Geometry check sheet. Reference: the model listing, model coordinates, mm. A direction names the side the tool comes from. Coordinates: 2 decimals unless noted, no trailing zeros. Loops run counter-clockwise (first coordinate to the right, second up) from the corner with the lowest first, then second, coordinate; pieces in that order, holes last. Notation, with made-up numbers: (-24.5, 49.5) - (22.5, 49.5) arc R30 cw to (22.5, 86.5) - close; hole circle Ø1 at (73, -34). An arc over 180 degrees is marked (long way). Write each question's results on one line, items separated by ' | '. Start each with the question number.
(1) Sectioned sample at B-B (z = 9.5). Enter the section's corners in (x, y), plus the area to 3 significant figures.
(2) Material ranges on probe 1 along Z at (x, y) = (-1.5, 15) (3 decimals); probe 2 along Z at (x, y) = (1.5, 9.5); probe 3 along Y at (x, z) = (-5.75, -13), recorded low to high.
(3) Sectioned sample at D-D (y = 10.5). Enter the section's corners in (x, z).
(4) Sectioned sample at A-A (x = 0.5). Enter the section's corners in (y, z) (3 decimals), plus the area to 3 significant figures.
(5) Go/stop test with flat-tipped pins: pin 1 Ø7 at (y, z) = (12, -0.5) entering from +X; pin 2 Ø6 at (x, z) = (0.5, 6.87) entering from -Y; pin 3 Ø7 at (y, z) = (11, -4) entering from -X. Record where each tip stops, or that it passes through.
(6) Sectioned sample at C-C (z = -1.5). Enter the section's corners in (x, y).
(7) Access from +Z, -Z, +X, -X, +Y, -Y to the whole of each face (thin tool, end or side, straight path). Record for faces 4 (the face through (13, 1, 0)), 5 (the face through (0.358, 9.098, -14.815)), 6 (the face through (0.64, 9.1, 13.32)), 7 (the face through (-5.95, 9, -1)), 8 (the face through (6.95, 9, -1)).
(8) Mould release check, pull along X, two halves, no side actions. Record for faces 1 (the face through (-13, 1, 0)), 2 (the face through (1.99, 8.11, 11.59)), 3 (the face through (0, 0, 0)): pulls with the +X half, pulls with the -X half, needs draft (parallel to the pull), parting line crosses it, or undercut.
from build123d import *

# Parameters (mm, degrees)
SKETCH_1_W          = 26
SKETCH_1_H          = 30.33
EXTRUDE_1_DEPTH     = 2
SKETCH_2_R          = 4.95
CUT_EXTRUDE_1_DEPTH = 21.07429264
EXTRUDE_START       = 14
SKETCH_3_R          = 4.95
EXTRUDE_2_DEPTH     = 14


with BuildPart() as part:
    # Эскиз1 → Бобышка-Вытянуть1 (new body)
    with BuildSketch(Plane(origin=(0, 0, 0), x_dir=(1, 0, 0), z_dir=(0, 1, 0))):
        Rectangle(SKETCH_1_W, SKETCH_1_H)
    extrude(amount=EXTRUDE_1_DEPTH)

    # Эскиз2 → Вырез-Вытянуть1 (cut, through all)
    with BuildSketch(Plane(origin=(0, 2, 0), x_dir=(1, 0, 0), z_dir=(0, 1, 0))):
        with Locations(Location((0.5, -6.870000865, 0), (0, 0, 270))):
            Circle(SKETCH_2_R)
        with Locations(Location((0.5, 8.367040316, 0), (0, 0, 270))):
            Circle(SKETCH_2_R)
    extrude(amount=-CUT_EXTRUDE_1_DEPTH, mode=Mode.SUBTRACT)

    # Эскиз3 → Бобышка-Вытянуть2 (add)
    with BuildSketch(Plane(origin=(0, 2, 0), x_dir=(1, 0, 0), z_dir=(0, 1, 0)).offset(EXTRUDE_START)):
        with BuildLine():
            Line((-5.95, -6.870000865), (-5.95, 8.367040316))
            ThreePointArc((-5.95, 8.367040316), (0.5, 14.817040316), (6.95, 8.367040316))
            Line((6.95, 8.367040316), (6.95, -6.870000865))
            ThreePointArc((6.95, -6.870000865), (0.5, -13.320000865), (-5.95, -6.870000865))
        make_face()
        with Locations(Location((0.5, -6.870000865, 0), (0, 0, 270))):
            Circle(SKETCH_3_R, mode=Mode.SUBTRACT)
        with Locations(Location((0.5, 8.367040316, 0), (0, 0, 270))):
            Circle(SKETCH_3_R, mode=Mode.SUBTRACT)
    extrude(amount=-EXTRUDE_2_DEPTH)


solid = part.part
Outcome:
1) outline: (-13, 0) - (-3.69, 0) - (-3.69, 16) - (-5.39, 16) - (-5.39, 2) - (-13, 2) - close; (4.69, 0) - (13, 0) - (13, 2) - (6.39, 2) - (6.39, 16) - (4.69, 16) - close | area: 82.7 mm2
2) probe 1: z = -14.499 to -12.895, -3.839 to 2.342, 11.398 to 13.002 | probe 2: z = -14.74 to -13.21, -3.52 to 2.02, 11.72 to 13.24 | probe 3: y = 0 to 2
3) outline: (-5.95, -8.37) arc R6.45 ccw to (6.95, -8.37) - (6.95, 6.87) arc R6.45 ccw to (-5.95, 6.87) - close; hole circle Ø9.9 at (0.5, -8.37); hole circle Ø9.9 at (0.5, 6.87)
4) outline: (0, -15.165) - (2, -15.165) - (2, -14.817) - (16, -14.817) - (16, -13.317) - (0, -13.317) - close; (0, -3.417) - (16, -3.417) - (16, 1.92) - (0, 1.92) - close; (0, 11.82) - (16, 11.82) - (16, 13.32) - (2, 13.32) - (2, 15.165) - (0, 15.165) - close | area: 138 mm2
5) pin 1: stops at x = 6.95 | pin 2: passes through | pin 3: stops at x = -5.95
6) outline: (-13, 0) - (13, 0) - (13, 2) - (6.95, 2) - (6.95, 16) - (-5.95, 16) - (-5.95, 2) - (-13, 2) - close
7) face 4: +Z, -Z, +X, +Y, -Y | face 5: -Z, +Y | face 6: +Z, +Y | face 7: +Z, -Z, -X, +Y | face 8: +Z, -Z, +X, +Y
8) face 1: pulls with the -X half | face 2: undercut | face 3: needs draft
